Design review of the part built by this model. Coordinates are the model's own, in mm. Coordinates: 2 decimals unless noted, no trailing zeros. Loops run counter-clockwise (first coordinate to the right, second up) from the corner with the lowest first, then second, coordinate; pieces in that order, holes last.
Q1. Add section A-A on x = -27.5. Give the boundary of the cut face in (y, z), and give its area (3 significant figures).
Q2. For P1, Ø1.5, axis at x = -5, y = -4.5, coming from the -Z side, flat-tipped, find the tip position at first contact; note if it passes through.
Q3. Wall thickness on probe 1 along X at (y, z) = (-59, 4.75); probe 2 along Y at (x, z) = (-30, 6.25): over which ranges is each line inside the solid? List them lowest first.
```python
from build123d import *

# Parameters (mm, degrees)
BOSS_EXTRUDE1_DEPTH = 7.62


with BuildPart() as part:
    # Sketch1 → Boss-Extrude1 (new body)
    with BuildSketch(Plane.XY):
        with BuildLine():
            Line((-22.606, -65.786), (22.606, -65.786))
            ThreePointArc((22.606, -65.786), (29.341192091, -62.996192091), (32.131, -56.261))
            Line((32.131, -56.261), (32.131, 56.261))
            ThreePointArc((32.131, 56.261), (29.341192091, 62.996192091), (22.606, 65.786))
            Line((22.606, 65.786), (-22.606, 65.786))
            ThreePointArc((-22.606, 65.786), (-29.341192091, 62.996192091), (-32.131, 56.261))
            Line((-32.131, 56.261), (-32.131, -56.261))
            ThreePointArc((-32.131, -56.261), (-29.341192091, -62.996192091), (-22.606, -65.786))
        make_face()
    extrude(amount=BOSS_EXTRUDE1_DEPTH)


solid = part.part
```
Entries:
1. outline: (-64.43, 0) - (64.43, 0) - (64.43, 7.62) - (-64.43, 7.62) - close
1. area: 982 mm2
2. P1: stops at z = 0
3. probe 1: x = -31.73 to 31.73
3. probe 2: y = -62.27 to 62.27
